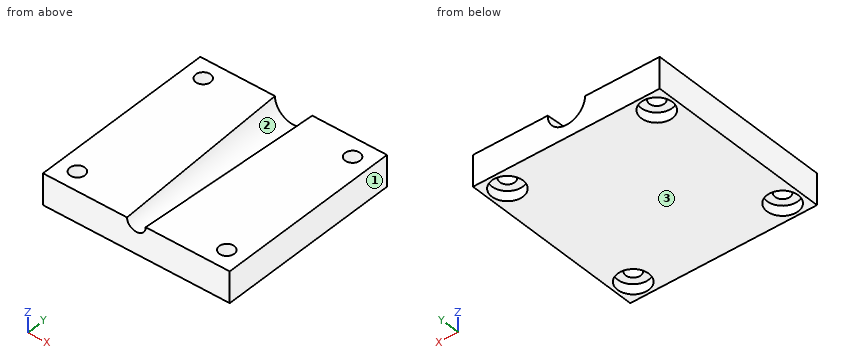
from build123d import *

# Parameters (mm, degrees)
SKETCH1_W                                        = 30
SKETCH1_H                                        = 30
BOSS_EXTRUDE1_DEPTH                              = 5
CBORE_FOR_M2_PAN_HEAD_MACHINE_SCREW1_D           = 2.4
CBORE_FOR_M2_PAN_HEAD_MACHINE_SCREW1_CBORE_D     = 5
CBORE_FOR_M2_PAN_HEAD_MACHINE_SCREW1_CBORE_DEPTH = 1.6


with BuildPart() as part:
    # Sketch1 → Boss-Extrude1 (new body)
    with BuildSketch(Plane.XY):
        with Locations((15, -15)):
            Rectangle(SKETCH1_W, SKETCH1_H)
    extrude(amount=BOSS_EXTRUDE1_DEPTH)

    # Sketch2 → Cut-Loft1 section 0
    with BuildSketch(Plane(origin=(0, 0, 0), x_dir=(1, 0, 0), z_dir=(0, 1, 0))):
        with BuildLine():
            Line((12, -5), (18, -5))
            ThreePointArc((18, -5), (15, -2), (12, -5))
        make_face()
    # Sketch3 → Cut-Loft1 section 1
    with BuildSketch(Plane.XZ.offset(30)):
        with BuildLine():
            Line((13.5, 5), (16.5, 5))
            ThreePointArc((16.5, 5), (15, 3.5), (13.5, 5))
        make_face()
    loft(mode=Mode.SUBTRACT)

    # CBORE for M2 Pan Head Machine Screw1 (through all)
    with Locations(Plane(origin=(0, 0, 0), x_dir=(-1, 0, 0), z_dir=(0, 0, -1))):
        with Locations((-27, -3), (-3, -3), (-3, -27), (-27, -27)):
            CounterBoreHole(CBORE_FOR_M2_PAN_HEAD_MACHINE_SCREW1_D / 2, CBORE_FOR_M2_PAN_HEAD_MACHINE_SCREW1_CBORE_D / 2, CBORE_FOR_M2_PAN_HEAD_MACHINE_SCREW1_CBORE_DEPTH)


solid = part.part
Geometry check sheet. Reference: the model listing, model coordinates, mm. Face numbers are marked on the shaded views. Round coordinates to 2 decimals unless told otherwise and drop trailing zeros. Order: outer loops, then holes, each group sorted by start corner. A loop starts at its lowest first (then second) coordinate and runs counter-clockwise, first axis right, second up. Notation, with made-up numbers: M 0,-21 L 52,-21 A28 cw 52,15 Z; hole C 61.5,-21.75 d6. An arc over 180 degrees is marked long. Answer in a Markdown table with one row per item.
(1) Sectioned sample at C-C, the plane x = 3. Record the cut outline in (y, z).
Responses:
| item | result |
|---|---|
| outline | M -30,0 L -29.5,0 L -29.5,1.6 L -28.2,1.6 L -28.2,5 L -30,5 Z; M -25.8,1.6 L -24.5,1.6 L -24.5,0 L -5.5,0 L -5.5,1.6 L -4.2,1.6 L -4.2,5 L -25.8,5 Z; M -1.8,1.6 L -0.5,1.6 L -0.5,0 L 0,0 L 0,5 L -1.8,5 Z |
(2) Scan lines: probe 1 along Y at (x, z) = (27, 0.7); probe 2 along Y at (x, z) = (3, 2.5); probe 3 along X at (y, z) = (-1.5, 3.2). Record each from-to range of solid material in increasing order. Write a range as from..to.
Responses:
| item | result |
|---|---|
| probe 1 | y = -30..-29.5, -24.5..-5.5, -0.5..0 |
| probe 2 | y = -30..-28.2, -25.8..-4.2, -1.8..0 |
| probe 3 | x = 0..12.69, 17.31..30 |
(3) Go/stop test with flat-tipped pins: P1, Ø4.5, axis at x = 3, y = -27, coming from the -Z side; P2, Ø4, axis at x = 3.5, y = -3.5, coming from the -Z side; P3, Ø1.4, axis at x = 27, y = -3, coming from the +Z side. Record where each tip stops, or that it passes through.
Responses:
| item | result |
|---|---|
| P1 | stops at z = 1.6 |
| P2 | stops at z = 0 |
| P3 | passes through |
(4) Sectioned sample at B-B, the plane z = 0.95. Record the cut outline in (x, y).
Responses:
| item | result |
|---|---|
| outline | M 0,-30 L 30,-30 L 30,0 L 0,0 Z; hole C 3,-27 d5; hole C 3,-3 d5; hole C 27,-27 d5; hole C 27,-3 d5 |
(5) Sectioned sample at A-A, the plane y = -3. Record the cut outline in (x, z).
Responses:
| item | result |
|---|---|
| outline | M 0,0 L 0.5,0 L 0.5,1.6 L 1.8,1.6 L 1.8,5 L 0,5 Z; M 4.2,1.6 L 5.5,1.6 L 5.5,0 L 24.5,0 L 24.5,1.6 L 25.8,1.6 L 25.8,5 L 17.85,5 A2.85 cw 12.15,5 L 4.2,5 Z; M 28.2,1.6 L 29.5,1.6 L 29.5,0 L 30,0 L 30,5 L 28.2,5 Z |
(6) Draft check along X on the marked faces 1, 2 and 3. Enter one of: released by +X, released by -X, zero draft, split by the parting line, or undercut.
Responses:
| item | result |
|---|---|
| face 1 | released by +X |
| face 2 | undercut |
| face 3 | zero draft |
(7) Sectioned sample at D-D, the plane y = -27. Record the cut outline in (x, z), and give its area (3 significant figures).
Responses:
| item | result |
|---|---|
| outline | M 0,0 L 0.5,0 L 0.5,1.6 L 1.8,1.6 L 1.8,5 L 0,5 Z; M 4.2,1.6 L 5.5,1.6 L 5.5,0 L 24.5,0 L 24.5,1.6 L 25.8,1.6 L 25.8,5 L 16.65,5 A1.65 cw 13.35,5 L 4.2,5 Z; M 28.2,1.6 L 29.5,1.6 L 29.5,0 L 30,0 L 30,5 L 28.2,5 Z |
| area | 113 mm² |
